Design review of the part built by this model. Coordinates are the model's own, in mm. Face numbers are marked on the shaded views. A direction names the side the tool comes from. Coordinates: 2 decimals unless noted, no trailing zeros. Write each loop counter-clockwise with the first axis right and the second up, starting at its lowest first coordinate (ties: lowest second). Pieces come first, ordered by that corner, then holes.
Q1. Take a section at B-B, the plane x = 1116. Write out the cut boundary in (y, z), plus the area to 3 significant figures.
Q2. For L1, parallel to Y at x = 144, z = 169.5; L2, parallel to Y at x = 828.5, z = -85.5; L3, parallel to X at y = 894, z = 400.5, list the stretches that pass through material, from the lowest coordinate up.
Q3. For the marked faces 4, 5 and 6, list the 3-axis set-ups (+Z, -Z, +X, -X, +Y, -Y) from which the entire face can be reached by the end or side of a thin tool; tool diameter is ignored.
Q4. Take a section at C-C, the plane z = -32. Write out the cut boundary in (x, y).
Q5. Take a section at A-A, the plane y = 1036. Write out the cut boundary in (x, z), plus the area to 3 significant figures.
Q6. For pin 1 Ø3 at (x, z) = (291, 329.5) entering from -Y; pin 2 Ø12 at (y, z) = (780, 57.5) entering from +X; pin 3 Ø1.5 at (x, z) = (1906.5, 226.5) entering from +Y; pin 4 Ø4 at (y, z) = (556.5, -191) entering from +X, all flat-tipped, find the tip position at first contact; note any pin that passes through.
Q7. Take a section at D-D, the plane y = 170. Write out the cut boundary in (x, z), plus the area to 3 significant figures.
Q8. The part is to be moulded in two halves that separate along Z. For the marked faces 1, 2 and 3, say which applies: released by +Z, released by -Z, zero draft, split by the parting line, or undercut.
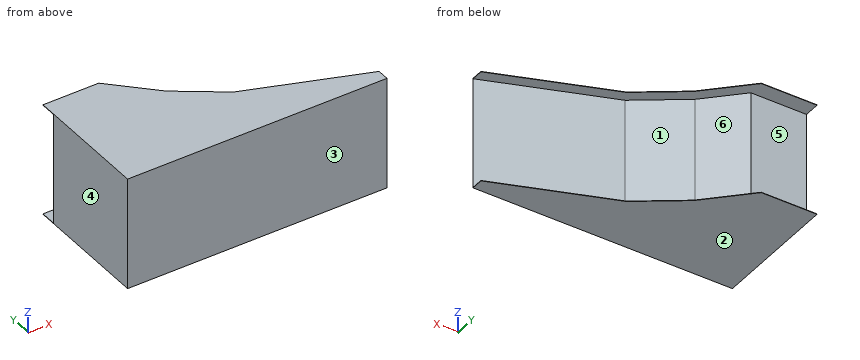
from build123d import *

# Parameters (mm, degrees)
AUFSATZ_LINEAR_AUSTRAGEN1_DEPTH = 500
AUFSATZ_LINEAR_AUSTRAGEN2_DEPTH = 4


with BuildPart() as part:
    # Skizze1 → Aufsatz-Linear austragen1 (new body, symmetric)
    with BuildSketch(Plane.XY):
        Polygon((0, 0), (0, 1000), (500, 1000), (800, 700), (1228.444402023, 400), (2327.435369805, 0), align=None)
    extrude(amount=AUFSATZ_LINEAR_AUSTRAGEN1_DEPTH, both=True)

    # Skizze3 → Aufsatz-Linear austragen2 (add)
    with BuildSketch(Plane.XY.offset(500)):
        Polygon((0, 0), (0, 1141.421356237), (500, 1141.421356237), (864.524295393, 776.897060844), (1275.017704404, 489.466481469), (2327.435369805, 106.417777248), (2327.435369805, 0), align=None)
    aufsatz_linear_austragen2 = extrude(amount=AUFSATZ_LINEAR_AUSTRAGEN2_DEPTH)

    # Spiegeln1: Aufsatz-Linear austragen2 across plane
    add(aufsatz_linear_austragen2.mirror(Plane(origin=(0, 0, 0), x_dir=(1, 0, 0), z_dir=(0, 0, -1))))


solid = part.part
Responses:
1. outline: (0, -504) - (600.81, -504) - (600.81, -500) - (478.73, -500) - (478.73, 500) - (600.81, 500) - (600.81, 504) - (0, 504) - close
1. area: 484,000 mm2
2. L1: y = 0 to 1000
2. L2: y = 0 to 680.04
2. L3: x = 0 to 606
3. face 4: +Z, -Z, -X, +Y, -Y
3. face 5: +X, -X, +Y
3. face 6: +X, +Y
4. outline: (0, 0) - (2327.44, 0) - (1228.44, 400) - (800, 700) - (500, 1000) - (0, 1000) - close
5. outline: (0, -504) - (605.42, -504) - (605.42, -500) - (0, -500) - close; (0, 500) - (605.42, 500) - (605.42, 504) - (0, 504) - close
5. area: 4,840 mm2
6. pin 1: stops at y = 0
6. pin 2: stops at x = 726
6. pin 3: stops at y = 153.48
6. pin 4: stops at x = 1007.8
7. outline: (0, -504) - (2152.74, -504) - (2152.74, -500) - (1860.36, -500) - (1860.36, 500) - (2152.74, 500) - (2152.74, 504) - (0, 504) - close
7. area: 1,880,000 mm2
8. face 1: undercut
8. face 2: released by -Z
8. face 3: zero draft
